```python
from build123d import *

# Parameters (mm, degrees)
SKETCH_1_W          = 168
SKETCH_1_H          = 25
EXTRUDE_1_DEPTH     = 40
SKETCH_2_R          = 25.5
CUT_EXTRUDE_1_DEPTH = 175.496418301
SKETCH_3_W          = 156
SKETCH_3_H          = 25
CUT_EXTRUDE_2_DEPTH = 8
CUT_EXTRUDE_3_DEPTH = 8
SKETCH_5_R          = 1.6
CUT_EXTRUDE_4_DEPTH = 175.496418301
CUT_EXTRUDE_5_DEPTH = 173.838074509
FILLET_2_R          = 1
FILLET_3_R          = 3
FILLET_4_R          = 3
FILLET_5_R          = 3


with BuildPart() as part:
    # Sketch 1 → Extrude 1 (new body)
    with BuildSketch(Plane.XY):
        with Locations((84, -12.5)):
            Rectangle(SKETCH_1_W, SKETCH_1_H)
    extrude(amount=EXTRUDE_1_DEPTH)

    # Sketch 2 → Cut-Extrude 1 (cut, through all)
    with BuildSketch(Plane.XY.offset(40)):
        with Locations((84, 10)):
            Circle(SKETCH_2_R)
    extrude(amount=-CUT_EXTRUDE_1_DEPTH, mode=Mode.SUBTRACT)

    # Sketch 3 → Cut-Extrude 2 (cut)
    with BuildSketch(Plane(origin=(0, 0, 0), x_dir=(-1, 0, 0), z_dir=(0, 0, -1))):
        with Locations((-84, -12.5)):
            Rectangle(SKETCH_3_W, SKETCH_3_H)
    extrude(amount=-CUT_EXTRUDE_2_DEPTH, mode=Mode.SUBTRACT)

    # Sketch 4 → Cut-Extrude 3 (cut)
    with BuildSketch(Plane.XY.offset(40)):
        with BuildLine():
            Line((162, 0), (107.457408211, 0))
            ThreePointArc((107.457408211, 0), (84, -15.5), (60.542591789, 0))
            Line((60.542591789, 0), (6, 0))
            Line((6, 0), (6, -25))
            Line((6, -25), (162, -25))
            Line((162, -25), (162, 0))
        make_face()
    extrude(amount=-CUT_EXTRUDE_3_DEPTH, mode=Mode.SUBTRACT)

    # Sketch 5 → Cut-Extrude 4 (cut, through all)
    with BuildSketch(Plane.ZY):
        with Locations(Location((4, -5, 0), (0, 0, 270))):
            Circle(SKETCH_5_R)
        with Locations(Location((4, -20, 0), (0, 0, 270))):
            Circle(SKETCH_5_R)
        with Locations(Location((36, -20, 0), (0, 0, 270))):
            Circle(SKETCH_5_R)
        with Locations(Location((36, -5, 0), (0, 0, 270))):
            Circle(SKETCH_5_R)
    extrude(amount=-CUT_EXTRUDE_4_DEPTH, mode=Mode.SUBTRACT)

    # Sketch 7 → Cut-Extrude 5 (cut, through all)
    with BuildSketch(Plane.XY.offset(32)):
        Polygon((37.542591789, -3), (57.542591789, -3), (65.042591789, -15.990381057), align=None)
        Polygon((24.034609426, -22), (59.034609426, -22), (35.263531583, -10.771077843), align=None)
        Polygon((11, -5), (11, -20), (26, -12.5), align=None)
        Polygon((157, -5), (157, -20), (142, -12.5), align=None)
        Polygon((132.736468417, -10.771077843), (143.965390574, -22), (108.965390574, -22), align=None)
        Polygon((110.457408211, -3), (102.957408211, -15.990381057), (130.457408211, -3), align=None)
    extrude(amount=-CUT_EXTRUDE_5_DEPTH, mode=Mode.SUBTRACT)

    # Fillet 2
    fillet_2_edges = [part.edges().sort_by_distance(p)[0] for p in [
        (11, -5, 20),
        (26, -12.5, 20),
        (11, -20, 20),
        (24.034609426, -22, 20),
        (35.263531583, -10.771077843, 20),
        (59.034609426, -22, 20),
        (108.965390574, -22, 20),
        (132.736468417, -10.771077843, 20),
        (143.965390574, -22, 20),
        (142, -12.5, 20),
        (157, -5, 20),
        (157, -20, 20),
        (110.457408211, -3, 20),
        (130.457408211, -3, 20),
        (102.957408211, -15.990381057, 20),
        (65.042591789, -15.990381057, 20),
        (37.542591789, -3, 20),
        (57.542591789, -3, 20),
    ]]
    fillet(fillet_2_edges, radius=FILLET_2_R)

    # Fillet 3
    fillet_3_edges = [part.edges().sort_by_distance(p)[0] for p in [
        (107.457408211, 0, 20),
        (60.542591789, 0, 20),
    ]]
    fillet(fillet_3_edges, radius=FILLET_3_R)

    # Fillet 4
    fillet_4_edges = [part.edges().sort_by_distance(p)[0] for p in [
        (3, 0, 0),
        (3, 0, 40),
        (3, -25, 0),
        (3, -25, 40),
    ]]
    fillet(fillet_4_edges, radius=FILLET_4_R)

    # Fillet 5
    fillet_5_edges = [part.edges().sort_by_distance(p)[0] for p in [
        (165, 0, 40),
        (165, -25, 0),
        (165, -25, 40),
        (165, 0, 0),
    ]]
    fillet(fillet_5_edges, radius=FILLET_5_R)


solid = part.part
```
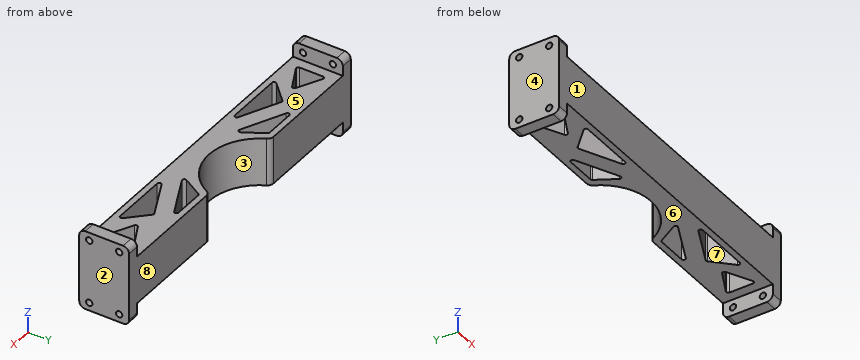
Check sheet for the modelled part. Datum: model origin and axes. Units: mm. Face numbers are marked on the shaded views. A direction names the side the tool comes from. Coordinates: 2 decimals unless noted, no trailing zeros. Write each loop counter-clockwise with the first axis right and the second up, starting at its lowest first coordinate (ties: lowest second). Pieces come first, ordered by that corner, then holes. Notation, with made-up numbers: M -0.5,-5.5 L 55.5,-5.5 A27 ccw 55.5,33.5 Z; hole C -5,16.25 d11. An arc over 180 degrees is marked long. Use one line per item in the form item = value.
Item 1: Sectioned sample at C-C, the plane x = 94. Record the cut outline in (y, z), and give its area (3 significant figures).
Answer below:
outline = M -25,8 L -13.46,8 L -13.46,32 L -25,32 Z
area = 277 mm^2
Item 2: Release check for a two-part mould opening along X. For the marked faces 1, 2 and 3 record: pulls with the +X half, pulls with the -X half, needs draft (parallel to the pull), parting line crosses it, or undercut.
Answer below:
face_1 = needs draft
face_2 = pulls with the +X half
face_3 = undercut
Item 3: Material ranges on L1, parallel to Z at x = 3.1, y = -5; L2, parallel to X at y = -21.25, z = 24.5; L3, parallel to X at y = -7, z = 4, recorded low to high. Write a range as from..to.
Answer below:
L1 = 0..2.4, 5.6..34.4, 37.6..40
L2 = 0..25.48, 55.54..112.46, 142.52..168
L3 = 0..6, 162..168
Item 4: Sectioned sample at A-A, the plane x = 135.5. Record the cut outline in (y, z).
Answer below:
outline = M -25,8 L -22,8 L -22,32 L -25,32 Z; M -13.53,8 L 0,8 L 0,32 L -13.53,32 Z
Item 5: Gauge pin test, flat ends, axial feed: pin 1 Ø4 at (y, z) = (-8.5, 35) entering from -X; pin 2 Ø12 at (x, z) = (99, 6) entering from +Y; pin 3 Ø12.5 at (x, y) = (82.5, -16.5) entering from +Z. Record the tip position at first contact, or that the pin passes through.
Answer below:
pin_1 = 0
pin_2 = -4.95
pin_3 = 32
Item 6: Sectioned sample at B-B, the plane x = 49. Record the cut outline in (y, z).
Answer below:
outline = M -25,8 L -22,8 L -22,32 L -25,32 Z; M -17.26,8 L -8.41,8 L -8.41,32 L -17.26,32 Z; M -3,8 L 0,8 L 0,32 L -3,32 Z
Item 7: Set-up check for the marked faces 4, 5, 6, 7 and 8: record each of +Z, -Z, +X, -X, +Y, -Y from which the full face is reachable in a straight line by a thin tool's end or side.
Answer below:
face_4 = +Z, -Z, -X, +Y, -Y
face_5 = +Z, +Y, -Y
face_6 = -Z, +Y, -Y
face_7 = +Z, -Z
face_8 = +Z, -Z, +X, -X, +Y
